```python
from build123d import *

# Parameters (mm, degrees)
ESBO_O1_R                = 12.2
RESSALTO_EXTRUS_O1_DEPTH = 6


with BuildPart() as part:
    # Esboço1 → Ressalto-extrusão1 (new body)
    with BuildSketch(Plane.XY):
        with BuildLine():
            Line((-94, 0), (-60, 0))
            Line((-60, 0), (-60, 6))
            Line((-60, 6), (-70, 6))
            Line((-70, 6), (-70, 86))
            Line((-70, 86), (70, 86))
            Line((70, 86), (70, 6))
            Line((70, 6), (60, 6))
            Line((60, 6), (60, 0))
            Line((60, 0), (94, 0))
            Line((94, 0), (40.861662232, -35.044161486))
            ThreePointArc((40.861662232, -35.044161486), (32.967231691, -38.734342211), (24.345307444, -40))
            Line((24.345307444, -40), (-24.345307444, -40))
            ThreePointArc((-24.345307444, -40), (-32.967231691, -38.734342211), (-40.861662232, -35.044161486))
            Line((-40.861662232, -35.044161486), (-94, 0))
        make_face()
        with Locations((0, -22)):
            Circle(ESBO_O1_R, mode=Mode.SUBTRACT)
        with BuildLine():
            Line((54, 60), (54, 25))
            ThreePointArc((54, 25), (51.071067812, 17.928932188), (44, 15))
            Line((44, 15), (-44, 15))
            ThreePointArc((-44, 15), (-51.071067812, 17.928932188), (-54, 25))
            Line((-54, 25), (-54, 60))
            ThreePointArc((-54, 60), (-51.071067812, 67.071067812), (-44, 70))
            Line((-44, 70), (44, 70))
            ThreePointArc((44, 70), (51.071067812, 67.071067812), (54, 60))
        make_face(mode=Mode.SUBTRACT)
    extrude(amount=RESSALTO_EXTRUS_O1_DEPTH)


solid = part.part
```
Can you work these out from the model? Positions are in its coordinate system, mm. A direction names the side the tool comes from. Coordinates: 2 decimals unless noted, no trailing zeros. Loops run counter-clockwise (first coordinate to the right, second up) from the corner with the lowest first, then second, coordinate; pieces in that order, holes last. Notation, with made-up numbers: (33.25, 48) -> (76.25, 48) arc R30 cw to (76.25, 87) -> close; hole circle Ø5 at (-14.75, 40). An arc over 180 degrees is marked (long way). Put each result on its own line as item: value. Start each with the question number.
Q1. I'm going to push flat-ended pins straight in: P1, Ø1.8, axis at y = 43.5, z = 1.5, coming from the -X side; P2, Ø1.8, axis at x = 64, z = 2, coming from the -Y side; P3, Ø3, axis at y = 41.5, z = 3, coming from the +X side. Where does each tip first touch, or does it pass through?
Q2. I want a section at B-B (x = 0). Write out the boundary of the cut face in (y, z).
Q3. I want a section at C-C (z = 1.4). Write out the boundary of the cut face in (x, y).
Q4. For faces 5 (the face through (1, 10, 6)), 6 (the face through (-70, 45, 3)), 7 (the face through (-50.99, 17.85, 2.96)), 8 (the face through (-77, 0, 3)), which set-ups out of +Z, -Z, +X, -X, +Y, -Y let a thin tool reach every point of the face, with its end or its side?
Q5. If I drill on line 1 (Y direction, x = 0, z = 3.6); line 2 (X direction, y = 32, z = 3.5); line 3 (X direction, y = 17, z = 0.6), over which ranges is the centre line in solid material (lowest first)? Write a range as [from, to].
Q6. Thinking about a two-plate mould opening in Y: for faces 1 (the face through (70, 47, 3)), 2 (the face through (-67.059, -17.767, 2.958)), 3 (the face through (60, 3, 3)), 4 (the face through (-51.15, 66.99, 2.96)), which applies, pulls with the +Y half, pulls with the -Y half, needs draft (parallel to the pull), parting line crosses it, or undercut?
Q7. I want a section at D-D (x = -48.5). Write out the boundary of the cut face in (y, z).
Q8. I want a section at A-A (y = 53.5). Write out the boundary of the cut face in (x, z).
Taken from the geometry:
1. P1: stops at x = -70
1. P2: stops at y = -20.38
1. P3: stops at x = 70
2. outline: (-40, 0) -> (-34.2, 0) -> (-34.2, 6) -> (-40, 6) -> close; (-9.8, 0) -> (15, 0) -> (15, 6) -> (-9.8, 6) -> close; (70, 0) -> (86, 0) -> (86, 6) -> (70, 6) -> close
3. outline: (-94, 0) -> (-40.86, -35.04) arc R30 ccw to (-24.35, -40) -> (24.35, -40) arc R30 ccw to (40.86, -35.04) -> (94, 0) -> (60, 0) -> (60, 6) -> (70, 6) -> (70, 86) -> (-70, 86) -> (-70, 6) -> (-60, 6) -> (-60, 0) -> close; hole (-54, 25) arc R10 ccw to (-44, 15) -> (44, 15) arc R10 ccw to (54, 25) -> (54, 60) arc R10 ccw to (44, 70) -> (-44, 70) arc R10 ccw to (-54, 60) -> close; hole circle Ø24.4 at (0, -22)
4. face 5: +Z, +X, -X, +Y, -Y
4. face 6: +Z, -Z, -X, +Y
4. face 7: +Z, -Z
4. face 8: +Z, -Z, -X
5. line 1: y = [-40, -34.2], [-9.8, 15], [70, 86]
5. line 2: x = [-70, -54], [54, 70]
5. line 3: x = [-70, -50], [50, 70]
6. face 1: needs draft
6. face 2: pulls with the -Y half
6. face 3: undercut
6. face 4: undercut
7. outline: (-30.01, 0) -> (16.07, 0) -> (16.07, 6) -> (-30.01, 6) -> close; (68.93, 0) -> (86, 0) -> (86, 6) -> (68.93, 6) -> close
8. outline: (-70, 0) -> (-54, 0) -> (-54, 6) -> (-70, 6) -> close; (54, 0) -> (70, 0) -> (70, 6) -> (54, 6) -> close
